```python
from build123d import *

# Parameters (mm, degrees)
F0_R     = 2.5019
F1_DEPTH = 5.6642


with BuildPart() as f1:
    # F0 (on Front) → F1 (new body)
    with BuildSketch(Plane.XZ):
        with BuildLine():
            Line((43.378084, -3.81), (43.839709, -3.81))
            ThreePointArc((43.839709, -3.81), (47.425881, 0), (43.839709, 3.81))
            Line((43.839709, 3.81), (43.378084, 3.81))
            Line((43.378084, 3.81), (-42.917735, 3.81))
            Line((-42.917735, 3.81), (-43.37936, 3.81))
            ThreePointArc((-43.37936, 3.81), (-46.965532, 0), (-43.37936, -3.81))
            Line((-43.37936, -3.81), (-42.917735, -3.81))
            Line((-42.917735, -3.81), (43.378084, -3.81))
        make_face()
        with Locations((-43.148547, 0)):
            Circle(F0_R, mode=Mode.SUBTRACT)
        with Locations((43.608896, 0)):
            Circle(F0_R, mode=Mode.SUBTRACT)
    extrude(amount=F1_DEPTH)


solid = f1.part
```
Part model, mm, in its own coordinate system. Give positions to 0.01 mm unless a question says otherwise; leave off trailing zeros. Loops run counter-clockwise (first coordinate to the right, second up) from the corner with the lowest first, then second, coordinate; pieces in that order, holes last. Notation, with made-up numbers: M 53.25,-39 L 101.25,-39 A31 cw 101.25,-15 Z; hole C 52,-28 d2. An arc over 180 degrees is marked long. Return JSON: item names as keys, results as strings.
1) Drill centre lines: line 1 (X direction, y = -2.2, z = -0.5); line 2 (X direction, y = -3.75, z = 2); line 3 (Z direction, x = -42, y = -5.05). Where is each one in solid material? Low to high.
Calculated:
{"line 1": "x = -46.93 to -45.6, -40.7 to 41.16, 46.06 to 47.39", "line 2": "x = -46.4 to -44.65, -41.65 to 42.11, 45.11 to 46.86", "line 3": "z = -3.81 to -2.22, 2.22 to 3.81"}
2) Saw through at B-B, the plane y = -1.45. List the corners of the cut face in (x, z).
Calculated:
{"outline": "M -43.38,-3.81 L 43.84,-3.81 A3.82 ccw 43.84,3.81 L -43.38,3.81 A3.82 ccw Z; hole C -43.15,0 d5; hole C 43.61,0 d5"}
3) Pull direction X, two halves, no side cores. Call faces 1 (the face through (-46.965, -2.792, 0.081)), 2 (the face through (-40.76, -2.79, 0.75)), 3 (the face through (0, -5.664, 0)), 4 (the face through (45.92, -2.79, -0.96)): released by +X, released by -X, zero draft, split by the parting line, or undercut.
Calculated:
{"face 1": "released by -X", "face 2": "undercut", "face 3": "zero draft", "face 4": "undercut"}
4) Saw through at A-A, the plane z = 0. List the corners of the cut face in (x, y), then the cut area to 3 significant figures.
Calculated:
{"outline": "M -46.97,-5.66 L -45.65,-5.66 L -45.65,0 L -46.97,0 Z; M -40.65,-5.66 L 41.11,-5.66 L 41.11,0 L -40.65,0 Z; M 46.11,-5.66 L 47.43,-5.66 L 47.43,0 L 46.11,0 Z", "area": "478 mm2"}
5) Flat gauge pins, fed straight in: pin 1 Ø1.5 at (y, z) = (-5, 3) entering from +X; pin 2 Ø4.5 at (x, z) = (-43.15, 0) entering from -Y. Where does each tip first touch, or does it go through?
Calculated:
{"pin 1": "stops at x = 46.69", "pin 2": "passes through"}
